from build123d import *

# Parameters (mm, degrees)
F1_DEPTH = 25.4
F2_R     = 1.524
F3_T     = -2.54


with BuildPart() as f1:
    # F0 (on Top) → F1 (new body)
    with BuildSketch(Plane.XY):
        with BuildLine():
            Line((47.625, 76.2), (-47.625, 76.2))
            ThreePointArc((-47.625, 76.2), (-52.115128, 74.340128), (-53.975, 69.85))
            Line((-53.975, 69.85), (-53.975, -69.85))
            ThreePointArc((-53.975, -69.85), (-52.115128, -74.340128), (-47.625, -76.2))
            Line((-47.625, -76.2), (47.625, -76.2))
            ThreePointArc((47.625, -76.2), (52.115128, -74.340128), (53.975, -69.85))
            Line((53.975, -69.85), (53.975, 69.85))
            ThreePointArc((53.975, 69.85), (52.115128, 74.340128), (47.625, 76.2))
        make_face()
    extrude(amount=F1_DEPTH)

    # F2
    f2_edges = [f1.edges().sort_by_distance(p)[0] for p in [
        (0, 76.2, 25.4),
    ]]
    fillet(f2_edges, radius=F2_R)

    # F3
    f3_openings = [f1.faces().sort_by_distance(p)[0] for p in [
        (0, 0, 0),
    ]]
    offset(amount=F3_T, openings=f3_openings)


solid = f1.part
Part model, mm, in its own coordinate system. A direction names the side the tool comes from. Coordinates: 2 decimals unless noted, no trailing zeros. Write each loop counter-clockwise with the first axis right and the second up, starting at its lowest first coordinate (ties: lowest second). Pieces come first, ordered by that corner, then holes. Notation, with made-up numbers: (47, 23.25) - (78, 23.25) arc R11 ccw to (78, 36.25) - close; hole circle Ø5 at (13, 32). An arc over 180 degrees is marked (long way). Put each result on its own line as item: value.
1. Band-saw the part on A-A (z = 12.5). Write the cut outline in (x, y) (3 decimals), then the cut area to 3 significant figures.
Final values:
outline: (-53.975, -69.85) arc R6.35 ccw to (-47.625, -76.2) - (47.625, -76.2) arc R6.35 ccw to (53.975, -69.85) - (53.975, 69.85) arc R6.35 ccw to (47.625, 76.2) - (-47.625, 76.2) arc R6.35 ccw to (-53.975, 69.85) - close; hole (-51.435, -69.85) arc R3.81 ccw to (-47.625, -73.66) - (47.625, -73.66) arc R3.81 ccw to (51.435, -69.85) - (51.435, 69.85) arc R3.81 ccw to (47.625, 73.66) - (-47.625, 73.66) arc R3.81 ccw to (-51.435, 69.85) - close
area: 1,270 mm²
2. Band-saw the part on C-C (x = -17). Write the cut outline in (y, z).
Final values:
outline: (-76.2, 0) - (-73.66, 0) - (-73.66, 22.86) - (73.66, 22.86) - (73.66, 0) - (76.2, 0) - (76.2, 23.88) arc R1.52 ccw to (74.68, 25.4) - (-74.68, 25.4) arc R1.52 ccw to (-76.2, 23.88) - close
3. Probe line 1 along X through (y, z) = (-44, 20.5) (3 decimals); line 2 along Y through (x, z) = (15, 6.75); line 3 along Z through (x, y) = (-5.5, -21.5). List the from-to ranges inside material, lowest first. Write a range as [from, to].
Final values:
line 1: x = [-53.975, -51.435], [51.435, 53.975]
line 2: y = [-76.2, -73.66], [73.66, 76.2]
line 3: z = [22.86, 25.4]
4. Two-plate mould, pull along X, no slides. Class faces 1 (the flat face through (-1, -73.66, 11)), 2 (the cylindrical face through (-52.065, 74.389, 11.771)), 3 (the flat face through (53.975, -1, 12)): +X half, -X half, draft (parallel to the pull), parting line (faces both ways), or undercut.
Final values:
face 1: undercut
face 2: -X half
face 3: +X half
5. Flat gauge pin, fed straight in: pin 1 Ø2 at (x, y) = (-0.5, 45.5) entering from -Z. Where does the tip first touch, or does it go through?
Final values:
pin 1: stops at z = 22.86
6. Band-saw the part on B-B (y = 52). Write the cut outline in (x, z) (3 decimals), then the cut area to 3 significant figures.
Final values:
outline: (-53.975, 0) - (-51.435, 0) - (-51.435, 22.86) - (51.435, 22.86) - (51.435, 0) - (53.975, 0) - (53.975, 23.876) arc R1.524 ccw to (52.451, 25.4) - (-52.451, 25.4) arc R1.524 ccw to (-53.975, 23.876) - close
area: 389 mm²
7. 3-axis set-ups, long thin cutter, end or side, ignore diameter. For faces 4 (the flat face through (-1, -76.2, 12)), 5 (the cylindrical face through (-50.289, 72.574, 11.27)): which of +Z, -Z, +X, -X, +Y, -Y reach the whole face in a straight line?
Final values:
face 4: +Z, -Z, +X, -X, -Y
face 5: -Z
